from build123d import *

# Parameters (mm, degrees)
SKETCH1_R           = 17
BOSS_EXTRUDE1_DEPTH = 2
CIRPATTERN1_COUNT   = 4


with BuildPart() as part:
    # Sketch1 → Boss-Extrude1 (new body)
    with BuildSketch(Plane.XY):
        Circle(SKETCH1_R)
        with BuildLine():
            Line((-1, 3.872983346), (-1, 5.002983346))
            Line((-1, 5.002983346), (1, 5.002983346))
            Line((1, 5.002983346), (1, 3.872983346))
            ThreePointArc((1, 3.872983346), (0, -4), (-1, 3.872983346))
        make_face(mode=Mode.SUBTRACT)
    extrude(amount=BOSS_EXTRUDE1_DEPTH)

    # Sketch4 → CSK for M2.5 Flat Head Machine Screw1 (revolve, cut)
    with BuildSketch(Plane(origin=(5, 5, 2), x_dir=(0, -1, 0), z_dir=(1, 0, 0))):
        Polygon((0, 0), (0, 2), (1.5, 2), (1.5, 1.25), (2.75, 0), align=None)
    csk_for_m2_5_flat_head_machine_screw1 = revolve(axis=Axis((5, 5, 8.35), (0, 0, -1)), mode=Mode.SUBTRACT)

    # CirPattern1: CSK for M2.5 Flat Head Machine Screw1 ×4 about axis
    cirpattern1_axis = Axis((0, 0, 0), (0, 0, 1))
    for i in range(1, CIRPATTERN1_COUNT):
        add(csk_for_m2_5_flat_head_machine_screw1.rotate(cirpattern1_axis, i * 360 / CIRPATTERN1_COUNT), mode=Mode.SUBTRACT)


solid = part.part
Can you work these out from the model? Positions are in its coordinate system, mm. A direction names the side the tool comes from. Round coordinates to 2 decimals unless told otherwise and drop trailing zeros. Write each loop counter-clockwise with the first axis right and the second up, starting at its lowest first coordinate (ties: lowest second). Pieces come first, ordered by that corner, then holes. Notation, with made-up numbers: (4.25, 25.25) -> (43.25, 25.25) arc R35 cw to (43.25, 59.25) -> close; hole circle Ø4 at (71, 35). An arc over 180 degrees is marked (long way). Use one line per item in the form item = value. Start each with the question number.
Q1. Which directions (+Z, -Z, +X, -X, +Y, -Y) give clear straight access to the entire face, cutting with the end or side of a thin tool? Please do faces 1 (the face through (0, 5.003, 1)), 2 (the face through (0, -7, 2)).
Q2. If I drill on probe 1 along X at (y, z) = (6, 0.8); probe 2 along X at (y, z) = (-4.5, 1.5); probe 3 along Y at (x, z) = (5, 0.5), over which ranges is the centre line in solid material (lowest first)? Write a range as [from, to].
Q3. Imagine slicing it at D-D (y = -5). Please give me the cut outline in (x, z), then the cut area to 3 significant figures.
Q4. I'm going to push flat-ended pins straight in: P1, Ø7, axis at x = 0, y = 0, coming from the +Z side; P2, Ø5, axis at x = 5, y = -5, coming from the +Z side. Where does each tip first touch, or does it pass through?
Q5. We'd pull the mould along X, two halves only. Please class faces 3 (the face through (3.5, -3.5, 0)), 4 (the face through (-1, 4.4, 1)), 5 (the face through (3.99, 6.11, 0.38)), 6 (the face through (9.139, 14.334, 0.986)): +X half, -X half, draft (parallel to the pull), parting line (faces both ways), or undercut.
Q6. Imagine slicing it at B-B (z = 0.35). Please give me the cut outline in (x, y).
Q7. Imagine slicing it at A-A (x = 0). Please give me the cut outline in (y, z).
Q8. Imagine slicing it at C-C (y = 0). Please give me the cut outline in (x, z).
Worked out:
q1.face_1 = +Z, -Z
q1.face_2 = +Z, +X, -X, +Y, -Y
q2.probe_1 = [-15.91, -6.18], [-3.82, 3.82], [6.18, 15.91]
q2.probe_2 = [-16.39, -7.19], [-2.81, 2.81], [7.19, 16.39]
q2.probe_3 = [-16.25, -6.5], [-3.5, 3.5], [6.5, 16.25]
q3.outline = (-16.25, 0) -> (-6.5, 0) -> (-6.5, 0.75) -> (-7.75, 2) -> (-16.25, 2) -> close; (-3.5, 0) -> (3.5, 0) -> (3.5, 0.75) -> (2.25, 2) -> (-2.25, 2) -> (-3.5, 0.75) -> close; (6.5, 0) -> (16.25, 0) -> (16.25, 2) -> (7.75, 2) -> (6.5, 0.75) -> close
q3.area = 49.9 mm^2
q4.P1 = through
q4.P2 = 1.75
q5.face_3 = draft
q5.face_4 = undercut
q5.face_5 = undercut
q5.face_6 = parting line
q6.outline = circle Ø34 at (0, 0); hole circle Ø3 at (-5, -5); hole circle Ø3 at (-5, 5); hole (-1, 3.87) arc R4 ccw (long way) to (1, 3.87) -> (1, 5) -> (-1, 5) -> close; hole circle Ø3 at (5, -5); hole circle Ø3 at (5, 5)
q7.outline = (-17, 0) -> (-4, 0) -> (-4, 2) -> (-17, 2) -> close; (5, 0) -> (17, 0) -> (17, 2) -> (5, 2) -> close
q8.outline = (-17, 0) -> (-4, 0) -> (-4, 2) -> (-17, 2) -> close; (4, 0) -> (17, 0) -> (17, 2) -> (4, 2) -> close
